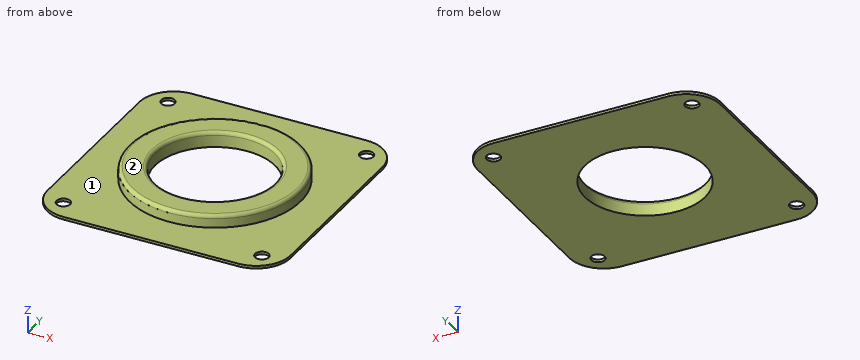
from build123d import *

# Parameters (mm, degrees)
SKETCH_1_W            = 71
SKETCH_1_H            = 71
EXTRUDE_1_DEPTH       = 0.8
SKETCH_2_W            = 25
SKETCH_2_H            = 3.7
HOLE_WIZARD_M30_1_D   = 35
HOLE_WIZARD_4_0_4_1_D = 4
FILLET_1_R            = 1
FILLET_2_R            = 10


with BuildPart() as part:
    # 草图1 → 凸台-拉伸1 (new body)
    with BuildSketch(Plane.XY.offset(1)):
        Rectangle(SKETCH_1_W, SKETCH_1_H)
    extrude(amount=-EXTRUDE_1_DEPTH)

    # 草图2 → 旋转1 (revolve)
    with BuildSketch(Plane.XZ, mode=Mode.PRIVATE) as revolve_1_sk:
        with Locations((12.5, 2.85)):
            Rectangle(SKETCH_2_W, SKETCH_2_H)
    revolve(revolve_1_sk.sketch.rotate(Axis((0, 0, 4.7), (0, 0, -1)), 180), axis=Axis((0, 0, 4.7), (0, 0, -1)))

    # M30 间隙孔1 (through all)
    with Locations(Plane.XY.offset(4.7)):
        with Locations((0, 0)):
            Hole(HOLE_WIZARD_M30_1_D / 2)

    # Ø4.0 (4) 直径孔1 (through all)
    with Locations(Plane.XY.offset(1)):
        with Locations((-29, 28.98), (-29, -29), (28.992753946, -28.992756445), (28.982756057, 28.982756057)):
            Hole(HOLE_WIZARD_4_0_4_1_D / 2)

    # 圆角1
    fillet_1_edges = [part.edges().sort_by_distance(p)[0] for p in [
        (25, 0, 4.7),
        (17.5, 0, 4.7),
    ]]
    fillet(fillet_1_edges, radius=FILLET_1_R)

    # 圆角2
    fillet_2_edges = [part.edges().sort_by_distance(p)[0] for p in [
        (35.5, 35.5, 0.6),
        (35.5, -35.5, 0.6),
        (-35.5, -35.5, 0.6),
        (-35.5, 35.5, 0.6),
    ]]
    fillet(fillet_2_edges, radius=FILLET_2_R)


solid = part.part
Design review of the part built by this model. Coordinates are the model's own, in mm. Face numbers are marked on the shaded views. A direction names the side the tool comes from. Coordinates: 2 decimals unless noted, no trailing zeros. Loops run counter-clockwise (first coordinate to the right, second up) from the corner with the lowest first, then second, coordinate; pieces in that order, holes last. Notation, with made-up numbers: M 39,3 L 51,3 A24 ccw 51,23 Z; hole C 71,80 d7. An arc over 180 degrees is marked long. Use one line per item in the form item = value.
(1) Clearance check with a flat-ended pin moving along its axis: P1, Ø2, axis at x = 10.5, y = 27, coming from the +Z side. State where the tip first meets the part, or that it passes through.
Return value:
P1 = 1
(2) Consider section C-C (y = -30). Write out the cut boundary in (x, z).
Return value:
outline = M -34.43,0.2 L -30.73,0.2 L -30.73,1 L -34.43,1 Z; M -27.27,0.2 L 27.26,0.2 L 27.26,1 L -27.27,1 Z; M 30.72,0.2 L 34.43,0.2 L 34.43,1 L 30.72,1 Z
(3) Consider section D-D (x = -29). Write out the cut boundary in (y, z).
Return value:
outline = M -34.87,0.2 L -31,0.2 L -31,1 L -34.87,1 Z; M -27,0.2 L 26.98,0.2 L 26.98,1 L -27,1 Z; M 30.98,0.2 L 34.87,0.2 L 34.87,1 L 30.98,1 Z
(4) Consider section A-A (y = 0). Write out the cut boundary in (x, z).
Return value:
outline = M -35.5,0.2 L -17.5,0.2 L -17.5,3.7 A1 ccw -18.5,4.7 L -24,4.7 A1 ccw -25,3.7 L -25,1 L -35.5,1 Z; M 17.5,0.2 L 35.5,0.2 L 35.5,1 L 25,1 L 25,3.7 A1 ccw 24,4.7 L 18.5,4.7 A1 ccw 17.5,3.7 Z
(5) For the marked faces 1 and 2, list the 3-axis set-ups (+Z, -Z, +X, -X, +Y, -Y) from which the entire face can be reached by the end or side of a thin tool; tool diameter is ignored.
Return value:
face_1 = +Z
face_2 = +Z, +X, -X, +Y, -Y
(6) For line 1 along Y through (x, z) = (-29, 0.8); line 2 along Y through (x, z) = (0, 2.1); line 3 along X through (y, z) = (9.5, 4.35), list the stretches that pass through material, from the lowest coordinate up. Write a range as from..to.
Return value:
line_1 = -34.87..-31, -27..26.98, 30.98..34.87
line_2 = -25..-17.5, 17.5..25
line_3 = -22.86..-14.98, 14.98..22.86
